Could you check a few things on this model? Use its own coordinates, in mm. Give positions to 0.01 mm unless a question says otherwise; leave off trailing zeros. Loops run counter-clockwise (first coordinate to the right, second up) from the corner with the lowest first, then second, coordinate; pieces in that order, holes last. Notation, with made-up numbers: (47, 35.25) - (75, 35.25) arc R21 cw to (75, 65.25) - close; hole circle Ø8 at (48, 4.5). An arc over 180 degrees is marked (long way). Write each question's results on one line, items separated by ' | '. Start each with the question number.
1) I want a section at D-D, the plane x = 8.5. Write out the boundary of the cut face in (y, z).
2) I want a section at C-C, the plane y = -19.05. Write out the boundary of the cut face in (x, z), and give its area (3 significant figures).
3) I want a section at B-B, the plane x = -38.5. Write out the boundary of the cut face in (y, z), and give its area (3 significant figures).
4) If I drill on probe 1 along Y at (x, z) = (0, 9.6); probe 2 along X at (y, z) = (55.5, 10.7); probe 3 along Y at (x, z) = (-38, 10.2), over which ranges is the centre line in solid material (lowest first)? Write a range as [from, to].
5) I want a section at A-A, the plane y = 6.35. Write out the boundary of the cut face in (x, z), and give its area (3 significant figures).
6) I'm going to push a flat-ended pin straight in: pin 1 (10 mm diameter, centred on x = -38.21, y = -19.05, fed in from -Z). Where does the tip first touch, or does it pass through?
7) If we mould it in two halves opening along Y, with no side actions, what happens to faces 1 (the face through (53.76, 58.39, 10.02)), 2 (the face through (1, -63.5, 10)), 3 (the face through (1, 1, 11.588))? For each: +Y half, -Y half, draft (parallel to the pull), parting line (faces both ways), or undercut.
from build123d import *
from build123d.topology import SkipClean

# Parameters (mm, degrees)
EXTRUDE1_START = 10
SKETCH1_W      = 63.5
SKETCH1_H      = 127
EXTRUDE1_DEPTH = 1.5875
SKETCH2_R      = 3.3528
SKETCH2_R_2    = 11.1125
SKETCH2_R_3    = 14.2875
SKETCH2_R_4    = 5.55625
EXTRUDE2_DEPTH = 90.858670283
FILLET1_R      = 0.508


with BuildPart() as part:
    # Sketch1 → Extrude1 (new, symmetric)
    with BuildSketch(Plane.XY.offset(EXTRUDE1_START)):
        with Locations((-31.75, 0)):
            Rectangle(SKETCH1_W, SKETCH1_H)
    extrude(amount=EXTRUDE1_DEPTH, both=True)

    # Sketch2 → Extrude2 (cut, through all)
    with BuildSketch(Plane.XY.offset(11.5875)):
        with Locations(Location((-55.5625, -55.5625, 0), (0, 0, 180))):
            Circle(SKETCH2_R)
        with Locations((0, 20.3454)):
            Circle(SKETCH2_R_2)
        with Locations((0, -20.3454)):
            Circle(SKETCH2_R_3)
        with Locations((-38.214808, 6.35)):
            Circle(SKETCH2_R_4)
        with Locations((-38.214808, -19.05)):
            Circle(SKETCH2_R_4)
        with Locations((-38.214808, 31.75)):
            Circle(SKETCH2_R_4)
        with Locations((-55.5625, 55.5625)):
            Circle(SKETCH2_R)
    extrude(amount=-EXTRUDE2_DEPTH, mode=Mode.SUBTRACT)

    # Fillet1
    fillet1_edges = [part.edges().sort_by_distance(p)[0] for p in [
        (-63.5, 63.5, 10),
        (-63.5, -63.5, 10),
    ]]
    fillet(fillet1_edges, radius=FILLET1_R)

    # Mirror1: part across plane


with BuildPart() as part_1:
    with SkipClean():  # the faces are left unmerged after this step: merging them gives an invalid solid
        add(part.part)
        add(part.part.mirror(Plane(origin=(0, 63.5, 11.5875), x_dir=(0, 0, 1), z_dir=(-1, 0, 0))))


solid = part_1.part
Answers:
1) outline: (-63.5, 8.41) - (-31.83, 8.41) - (-31.83, 11.59) - (-63.5, 11.59) - close; (-8.86, 8.41) - (13.19, 8.41) - (13.19, 11.59) - (-8.86, 11.59) - close; (27.5, 8.41) - (63.5, 8.41) - (63.5, 11.59) - (27.5, 11.59) - close
2) outline: (-63.5, 8.41) - (-43.77, 8.41) - (-43.77, 11.59) - (-63.5, 11.59) - close; (-32.66, 8.41) - (-14.23, 8.41) - (-14.23, 11.59) - (-32.66, 11.59) - close; (14.23, 8.41) - (32.66, 8.41) - (32.66, 11.59) - (14.23, 11.59) - close; (43.77, 8.41) - (63.5, 8.41) - (63.5, 11.59) - (43.77, 11.59) - close | area: 242 mm2
3) outline: (-63.5, 8.41) - (-24.6, 8.41) - (-24.6, 11.59) - (-63.5, 11.59) - close; (-13.5, 8.41) - (0.8, 8.41) - (0.8, 11.59) - (-13.5, 11.59) - close; (11.9, 8.41) - (26.2, 8.41) - (26.2, 11.59) - (11.9, 11.59) - close; (37.3, 8.41) - (63.5, 8.41) - (63.5, 11.59) - (37.3, 11.59) - close | area: 298 mm2
4) probe 1: y = [-63.5, -34.63], [-6.06, 9.23], [31.46, 63.5] | probe 2: x = [-63.5, -58.91], [-52.21, 52.21], [58.91, 63.5] | probe 3: y = [-63.5, -24.6], [-13.5, 0.8], [11.9, 26.2], [37.3, 63.5]
5) outline: (-63.5, 8.41) - (-43.77, 8.41) - (-43.77, 11.59) - (-63.5, 11.59) - close; (-32.66, 8.41) - (32.66, 8.41) - (32.66, 11.59) - (-32.66, 11.59) - close; (43.77, 8.41) - (63.5, 8.41) - (63.5, 11.59) - (43.77, 11.59) - close | area: 333 mm2
6) pin 1: passes through
7) face 1: undercut | face 2: -Y half | face 3: draft
